Check sheet for the modelled part. Datum: model origin and axes. Units: mm. Round coordinates to 2 decimals unless told otherwise and drop trailing zeros. Loops run counter-clockwise (first coordinate to the right, second up) from the corner with the lowest first, then second, coordinate; pieces in that order, holes last. Notation, with made-up numbers: (34, 68.5) - (44, 68.5) arc R22 ccw to (44, 78.5) - close; hole circle Ø8 at (0.5, 36). An arc over 180 degrees is marked (long way). Return JSON: item names as keys, results as strings.
from build123d import *

# Parameters (mm, degrees)
F1_R     = 1.75
F1_R_2   = 13.5
F2_DEPTH = 2.5


with BuildPart() as f2:
    # F1 (on Top) → F2 (new body)
    with BuildSketch(Plane.XY):
        with BuildLine():
            Line((10.2372021925, 69.3784194525), (9.8985145849, 69.2028852716))
            ThreePointArc((9.8985145849, 69.2028852716), (5.955561629, 65.5199035219), (4.5, 60.324465819))
            Line((4.5, 60.324465819), (4.5, 40))
            Line((4.5, 40), (4.5, 19.675534181))
            ThreePointArc((4.5, 19.675534181), (5.955561629, 14.4800964781), (9.8985145849, 10.7971147284))
            Line((9.8985145849, 10.7971147284), (10.2372021925, 10.6215805475))
            ThreePointArc((10.2372021925, 10.6215805475), (12.470586525, 9.7844404555), (14.8386876076, 9.5))
            Line((14.8386876076, 9.5), (15.5546120462, 9.5))
            ThreePointArc((15.5546120462, 9.5), (17.9366290245, 9.7878429216), (20.1815166575, 10.634800977))
            Line((20.1815166575, 10.634800977), (29.1640234003, 15.322930568))
            ThreePointArc((29.1640234003, 15.322930568), (31.4089110333, 16.1698886233), (33.7909280117, 16.457731545))
            Line((33.7909280117, 16.457731545), (56.8851493299, 16.457731545))
            ThreePointArc((56.8851493299, 16.457731545), (58.5333421059, 16.3209693791), (60.1364527991, 15.9144236596))
            Line((60.1364527991, 15.9144236596), (74.8714324464, 10.8483931845))
            ThreePointArc((74.8714324464, 10.8483931845), (78.7421893122, 10.3242898655), (82.518433429, 11.3230007209))
            Line((82.518433429, 11.3230007209), (86.1698560542, 13.1099522035))
            ThreePointArc((86.1698560542, 13.1099522035), (88.830601645, 15.0063744472), (90.7380024689, 17.6592608982))
            Line((90.7380024689, 17.6592608982), (96.1243657197, 28.5514243616))
            ThreePointArc((96.1243657197, 28.5514243616), (97.6717100474, 32.8647106004), (98.1966778636, 37.4169761286))
            Line((98.1966778636, 37.4169761286), (98.1966778636, 40))
            Line((98.1966778636, 40), (98.1966778636, 42.5830238714))
            ThreePointArc((98.1966778636, 42.5830238714), (97.6717100474, 47.1352893996), (96.1243657197, 51.4485756384))
            Line((96.1243657197, 51.4485756384), (90.7380024689, 62.3407391018))
            ThreePointArc((90.7380024689, 62.3407391018), (88.830601645, 64.9936255528), (86.1698560542, 66.8900477965))
            Line((86.1698560542, 66.8900477965), (82.518433429, 68.6769992791))
            ThreePointArc((82.518433429, 68.6769992791), (78.7421893122, 69.6757101345), (74.8714324464, 69.1516068155))
            Line((74.8714324464, 69.1516068155), (60.1364527991, 64.0855763404))
            ThreePointArc((60.1364527991, 64.0855763404), (58.5333421059, 63.6790306209), (56.8851493299, 63.542268455))
            Line((56.8851493299, 63.542268455), (33.7909280117, 63.542268455))
            ThreePointArc((33.7909280117, 63.542268455), (31.4089110333, 63.8301113767), (29.1640234003, 64.677069432))
            Line((29.1640234003, 64.677069432), (20.1815166575, 69.365199023))
            ThreePointArc((20.1815166575, 69.365199023), (17.9366290245, 70.2121570784), (15.5546120462, 70.5))
            Line((15.5546120462, 70.5), (14.8386876076, 70.5))
            ThreePointArc((14.8386876076, 70.5), (12.470586525, 70.2155595445), (10.2372021925, 69.3784194525))
        make_face()
        with Locations((14.5, 17)):
            Circle(F1_R, mode=Mode.SUBTRACT)
        with Locations((39.3913947046, 23)):
            Circle(F1_R, mode=Mode.SUBTRACT)
        with Locations((50, 23.5)):
            Circle(F1_R, mode=Mode.SUBTRACT)
        with BuildLine():
            ThreePointArc((27.2737251007, 51.9557933746), (29.1278270669, 51.9557933746), (30.6278270669, 50.8659795825))
            Line((30.6278270669, 50.8659795825), (37.2412703927, 41.7633557569))
            ThreePointArc((37.2412703927, 41.7633557569), (37.8142194096, 40), (37.2412703927, 38.2366442431))
            Line((37.2412703927, 38.2366442431), (30.6278270669, 29.1340204175))
            ThreePointArc((30.6278270669, 29.1340204175), (29.1278270669, 28.0442066254), (27.2737251007, 28.0442066254))
            Line((27.2737251007, 28.0442066254), (16.5729490169, 31.52109954))
            ThreePointArc((16.5729490169, 31.52109954), (15.0729490169, 32.6109133321), (14.5, 34.3742690889))
            Line((14.5, 34.3742690889), (14.5, 45.6257309111))
            ThreePointArc((14.5, 45.6257309111), (15.0729490169, 47.3890866679), (16.5729490169, 48.47890046))
            Line((16.5729490169, 48.47890046), (27.2737251007, 51.9557933746))
        make_face(mode=Mode.SUBTRACT)
        with Locations((45, 28.5)):
            Circle(F1_R, mode=Mode.SUBTRACT)
        with Locations((80, 18)):
            Circle(F1_R, mode=Mode.SUBTRACT)
        with Locations((85, 28.5)):
            Circle(F1_R, mode=Mode.SUBTRACT)
        with Locations((45, 51.5)):
            Circle(F1_R, mode=Mode.SUBTRACT)
        with Locations((14.5, 63)):
            Circle(F1_R, mode=Mode.SUBTRACT)
        with Locations((39.3913947046, 57)):
            Circle(F1_R, mode=Mode.SUBTRACT)
        with Locations((50, 56.5)):
            Circle(F1_R, mode=Mode.SUBTRACT)
        with Locations((65.432921052, 40)):
            Circle(F1_R_2, mode=Mode.SUBTRACT)
        with Locations((85, 51.5)):
            Circle(F1_R, mode=Mode.SUBTRACT)
        with Locations((80, 62)):
            Circle(F1_R, mode=Mode.SUBTRACT)
    extrude(amount=F2_DEPTH)


solid = f2.part
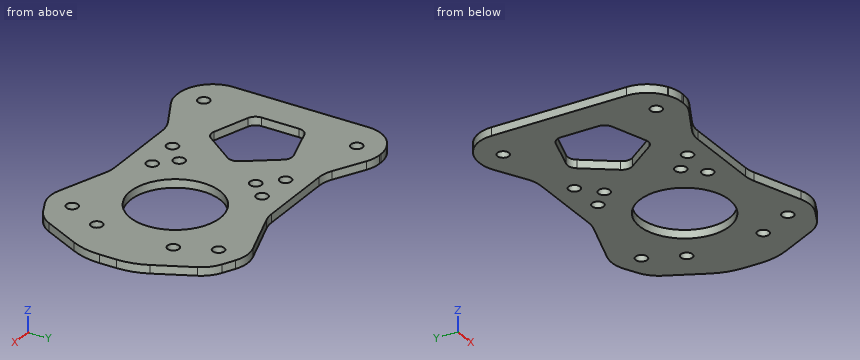
Q1. Sectioned sample at A-A (y = 40). Enter the section's corners in (x, z).
Answer key:
{"outline": "(4.5, 0) - (14.5, 0) - (14.5, 2.5) - (4.5, 2.5) - close; (37.81, 0) - (51.93, 0) - (51.93, 2.5) - (37.81, 2.5) - close; (78.93, 0) - (98.2, 0) - (98.2, 2.5) - (78.93, 2.5) - close"}
Q2. Depth check by flat-ended pin: P1, Ø10, axis at x = 38.5, y = 28, coming from the -Z side; P2, Ø1.2, axis at x = 40.5, z = 1.5, coming from the +Y side; P3, Ø1.5, axis at x = 32, z = 1.5, coming from the +Y side. Enter the tip coordinate at first touch or a pass-through.
Answer key:
{"P1": "stops at z = 0", "P2": "stops at y = 63.54", "P3": "stops at y = 63.87"}
Q3. Sectioned sample at D-D (z = 1.7). State how many separate pieces and enclosed holes the cut face has, plus the area to 3 significant figures.
Answer key:
{"separate pieces": "1", "enclosed holes": "14", "area": "3,640 mm²"}
Q4. Sectioned sample at B-B (x = 50). Enter the section's corners in (y, z), plus the area to 3 significant figures.
Answer key:
{"outline": "(16.46, 0) - (21.75, 0) - (21.75, 2.5) - (16.46, 2.5) - close; (25.25, 0) - (54.75, 0) - (54.75, 2.5) - (25.25, 2.5) - close; (58.25, 0) - (63.54, 0) - (63.54, 2.5) - (58.25, 2.5) - close", "area": "100 mm²"}
Q5. Scan lines: probe 1 along Y at (x, z) = (45, 1.8); probe 2 along X at (y, z) = (22, 1.15); probe 3 along Y at (x, z) = (50.5, 1.15). Record each from-to range of solid material in increasing order. Write a range as [from, to].
Answer key:
{"probe 1": "y = [16.46, 26.75], [30.25, 49.75], [53.25, 63.54]", "probe 2": "x = [4.5, 37.96], [40.83, 49.1], [50.9, 92.88]", "probe 3": "y = [16.46, 21.82], [25.18, 54.82], [58.18, 63.54]"}
Q6. Sectioned sample at C-C (x = 64.5). Enter the section's corners in (y, z), plus the area to 3 significant figures.
Answer key:
{"outline": "(14.41, 0) - (26.53, 0) - (26.53, 2.5) - (14.41, 2.5) - close; (53.47, 0) - (65.59, 0) - (65.59, 2.5) - (53.47, 2.5) - close", "area": "60.6 mm²"}
